Can you work these out from the model? Positions are in its coordinate system, mm. Face numbers are marked on the shaded views. A direction names the side the tool comes from. Give positions to 0.01 mm unless a question says otherwise; leave off trailing zeros. Order: outer loops, then holes, each group sorted by start corner. A loop starts at its lowest first (then second) coordinate and runs counter-clockwise, first axis right, second up. Notation, with made-up numbers: M 56.25,-15 L 68.25,-15 A19 ccw 68.25,-3 Z; hole C 1.25,42 d7. An arc over 180 degrees is marked long. Use one line per item in the form item = value. Start each with the question number.
1. I want a section at D-D, the plane y = 7. List the corners of the cut face in (x, z) for me, and give its area (3 significant figures).
2. We'd pull the mould along X, two halves only. Please class the marked faces 1, 2 and 3: +X half, -X half, draft (parallel to the pull), parting line (faces both ways), or undercut.
3. I want a section at C-C, the plane x = 0. List the corners of the cut face in (y, z) for me, and give its area (3 significant figures).
4. I want a section at B-B, the plane y = 3.5. Count the separate pieces of the cut face and the enclosed holes in it, and give its area (3 significant figures).
5. Will these pins go through, and if not, where does the flat tip stop? P1, Ø5.5, axis at y = 2, z = 2, coming from the -X side; P2, Ø0.8, axis at y = 4.5, z = -2.5, coming from the +X side; P3, Ø2, axis at y = 1.5, z = -3.5, coming from the +X side; P4, Ø3.5, axis at x = -11, z = 1, coming from the +Y side.
6. I want a section at A-A, the plane y = 5.5. List the corners of the cut face in (x, z) for me, and give its area (3 significant figures).
7. For the marked faces 4, 5 and 6, which set-ups out of +Z, -Z, +X, -X, +Y, -Y let a thin tool reach every point of the face, with its end or its side?
8. I need wall thicknesses on L1, parallel to X at y = 3.1, z = 0; L2, parallel to X at y = 5, z = 2.25; L3, parallel to Y at x = 10.5, z = -2.75. Which ranges of each line are inside material? Lowest first, please.
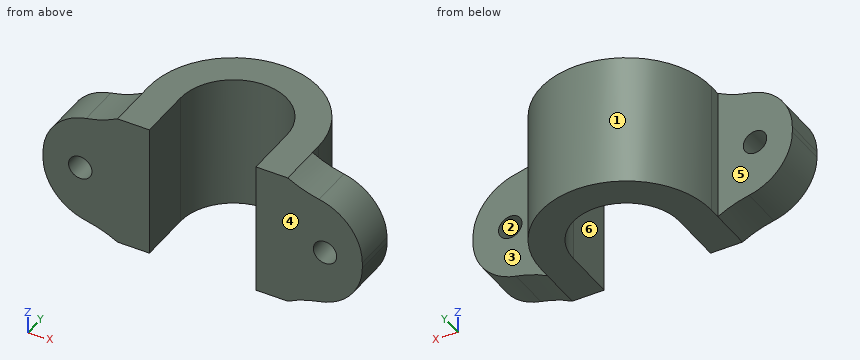
```python
from build123d import *

# Parameters (mm, degrees)
BOSS_EXTRUDE1_DEPTH = 6.25
BOSS_EXTRUDE4_REACH = 29.149
SKETCH5_W           = 10
SKETCH5_H           = 4
FILLET1_R           = 10
FILLET2_R           = 5
SKETCH7_R           = 1.1
CUT_EXTRUDE2_DEPTH  = 19.575858103
FILLET6_R           = 10
FILLET7_R           = 5


with BuildPart() as part:
    # Sketch1 → Boss-Extrude1 (new, symmetric)
    with BuildSketch(Plane.XY):
        with BuildLine():
            Line((5, 5), (5, 0))
            Line((5, 0), (8, 0))
            Line((8, 0), (8, 5))
            ThreePointArc((8, 5), (0, 13), (-8, 5))
            Line((-8, 5), (-8, 0))
            Line((-8, 0), (-5, 0))
            Line((-5, 0), (-5, 5))
            ThreePointArc((-5, 5), (0, 10), (5, 5))
        make_face()
    extrude(amount=BOSS_EXTRUDE1_DEPTH, both=True)

    # Sketch5 → Boss-Extrude4 (add, up to next)
    with BuildSketch(Plane(origin=(-15, 0, 0), x_dir=(0, 0, -1), z_dir=(1, 0, 0)), mode=Mode.PRIVATE) as boss_extrude4_sk1:
        with Locations((0, 2)):
            Rectangle(SKETCH5_W, SKETCH5_H)
    boss_extrude4_tool1 = extrude(boss_extrude4_sk1.sketch, amount=BOSS_EXTRUDE4_REACH, mode=Mode.PRIVATE) - part.part
    boss_extrude4 = boss_extrude4_tool1.solids().sort_by_distance((-15, 2, 0))[0]
    add(boss_extrude4)

    # Fillet1
    # the kernel refuses this fillet: 10 mm, written as the material it adds along each edge
    with BuildSketch(Plane(origin=(-8, 0, -5), x_dir=(0, 0, -1), z_dir=(0, 1, 0)), Plane(origin=(-8, 4, 5), x_dir=(0, 0, 1), z_dir=(0, -1, 0))) as fillet1_piece_1:
        with BuildLine():
            CenterArc((10, 4.841229183), FILLET1_R, 180, 28.955024372)
            Line((0, 4.841229183), (-0.2, 4.841229183))
            Line((-0.2, 4.841229183), (-0.2, 0))
            Line((-0.2, 0), (0, -0.2))
            ThreePointArc((0, -0.2), (0.625, -0.2), (1.075, -0.096824584))
            Line((1.075, -0.096824584), (1.25, 0))
        make_face()
    extrude(amount=4)

    # Fillet2
    fillet2_edges = [part.edges().sort_by_distance(p)[0] for p in [
        (-15, 2, -5),
        (-15, 2, 5),
    ]]
    fillet(fillet2_edges, radius=FILLET2_R)

    # Sketch7 → Cut-Extrude2 (cut, through all)
    with BuildSketch(Plane(origin=(0, 4, 0), x_dir=(1, 0, 0), z_dir=(0, 1, 0))):
        with Locations(Location((-11.5, 0, 0), (0, 0, 270))):
            Circle(SKETCH7_R)
    cut_extrude2 = extrude(amount=-CUT_EXTRUDE2_DEPTH, mode=Mode.SUBTRACT)

    # Mirror6: Boss-Extrude4 across plane
    add(boss_extrude4.mirror(Plane(origin=(0, 0, 0), x_dir=(0, 0, 1), z_dir=(1, 0, 0))))

    # Mirror7: Cut-Extrude2 across plane
    add(cut_extrude2.mirror(Plane(origin=(0, 0, 0), x_dir=(0, 0, 1), z_dir=(1, 0, 0))), mode=Mode.SUBTRACT)

    # Fillet6
    # the kernel refuses this fillet: 10 mm, written as the material it adds along each edge
    with BuildSketch(Plane(origin=(8, 4, 5), x_dir=(0, 0, 1), z_dir=(0, -1, 0)), Plane(origin=(8, 0, -5), x_dir=(0, 0, -1), z_dir=(0, 1, 0))) as fillet6_piece_1:
        with BuildLine():
            CenterArc((10, -4.841229183), FILLET6_R, 151.044975628, 28.955024372)
            Line((0, -4.841229183), (-0.2, -4.841229183))
            Line((-0.2, -4.841229183), (-0.2, 0))
            Line((-0.2, 0), (0, 0.2))
            ThreePointArc((0, 0.2), (0.625, 0.2), (1.075, 0.096824584))
            Line((1.075, 0.096824584), (1.25, 0))
        make_face()
    extrude(amount=4)

    # Fillet7
    fillet7_edges = [part.edges().sort_by_distance(p)[0] for p in [
        (15, 2, 5),
        (15, 2, -5),
    ]]
    fillet(fillet7_edges, radius=FILLET7_R)


solid = part.part
```
Check result:
q1.outline = M -7.75,-6.25 L -4.58,-6.25 L -4.58,6.25 L -7.75,6.25 Z; M 4.58,-6.25 L 7.75,-6.25 L 7.75,6.25 L 4.58,6.25 Z
q1.area = 79.1 mm2
q2.face_1 = parting line
q2.face_2 = undercut
q2.face_3 = draft
q3.outline = M 10,-6.25 L 13,-6.25 L 13,6.25 L 10,6.25 Z
q3.area = 37.5 mm2
q4.separate_pieces = 2
q4.enclosed_holes = 2
q4.area = 198 mm2
q5.P1 = -15
q5.P2 = 8
q5.P3 = 14.48
q5.P4 = 4
q6.outline = M -7.98,-6.25 L -4.97,-6.25 L -4.97,6.25 L -7.98,6.25 Z; M 4.97,-6.25 L 7.98,-6.25 L 7.98,6.25 L 4.97,6.25 Z
q6.area = 75.2 mm2
q7.face_4 = +Z, -Z, +X, -X, -Y
q7.face_5 = +Z, -Z, -X, +Y
q7.face_6 = +Z, -Z, -Y
q8.L1 = -15 to -12.6, -10.4 to -5, 5 to 10.4, 12.6 to 15
q8.L2 = -8 to -5, 5 to 8
q8.L3 = 0 to 4
